```python
from build123d import *

# Parameters (mm, degrees)
SKETCH1_W           = 203.2
SKETCH1_H           = 101.6
BOSS_EXTRUDE2_DEPTH = 203.2
FILLET3_R           = 20
FILLET4_R           = 20
FILLET5_R           = 20
FILLET6_R           = 20
SKETCH2_W           = 152.4
SKETCH2_H           = 152.4
CUT_EXTRUDE1_DEPTH  = 88.9


with BuildPart() as part:
    # Sketch1 → Boss-Extrude2 (new body)
    with BuildSketch(Plane.XY):
        with Locations((101.6, 50.8)):
            Rectangle(SKETCH1_W, SKETCH1_H)
    extrude(amount=BOSS_EXTRUDE2_DEPTH)

    # Fillet3
    fillet3_edges = [part.edges().sort_by_distance(p)[0] for p in [
        (0, 50.8, 0),
    ]]
    fillet(fillet3_edges, radius=FILLET3_R)

    # Fillet4
    fillet4_edges = [part.edges().sort_by_distance(p)[0] for p in [
        (203.2, 50.8, 0),
    ]]
    fillet(fillet4_edges, radius=FILLET4_R)

    # Fillet5
    fillet5_edges = [part.edges().sort_by_distance(p)[0] for p in [
        (0, 50.8, 203.2),
    ]]
    fillet(fillet5_edges, radius=FILLET5_R)

    # Fillet6
    fillet6_edges = [part.edges().sort_by_distance(p)[0] for p in [
        (203.2, 50.8, 203.2),
    ]]
    fillet(fillet6_edges, radius=FILLET6_R)

    # Sketch2 → Cut-Extrude1 (cut)
    with BuildSketch(Plane.XZ):
        with Locations((100, 100)):
            Rectangle(SKETCH2_W, SKETCH2_H)
    extrude(amount=-CUT_EXTRUDE1_DEPTH, mode=Mode.SUBTRACT)


solid = part.part
```
Can you work these out from the model? Positions are in its coordinate system, mm. A direction names the side the tool comes from. Round coordinates to 2 decimals unless told otherwise and drop trailing zeros. Order: outer loops, then holes, each group sorted by start corner. A loop starts at its lowest first (then second) coordinate and runs counter-clockwise, first axis right, second up.
(1) If we section it at A-A (z = 52.5): Please give me the cut outline in (x, y), plus the area to 3 significant figures.
Results are:
outline: (0, 0) - (23.8, 0) - (23.8, 88.9) - (176.2, 88.9) - (176.2, 0) - (203.2, 0) - (203.2, 101.6) - (0, 101.6) - close
area: 7,100 mm2
(2) We'd pull the mould along Z, two halves only. Please class faces 1 (the face through (99, 44, 176.2)), 2 (the face through (5.703, 51.511, 6.014)), 3 (the face through (197.186, 51.511, 197.497)): +Z half, -Z half, draft (parallel to the pull), parting line (faces both ways), or undercut.
Results are:
face 1: undercut
face 2: -Z half
face 3: +Z half
(3) If we section it at C-C (y = 53): Please give me the cut outline in (x, z).
Results are:
outline: (0, 20) arc R20 ccw to (20, 0) - (183.2, 0) arc R20 ccw to (203.2, 20) - (203.2, 183.2) arc R20 ccw to (183.2, 203.2) - (20, 203.2) arc R20 ccw to (0, 183.2) - close; hole (23.8, 23.8) - (176.2, 23.8) - (176.2, 176.2) - (23.8, 176.2) - close
(4) If I drill on L1, parallel to X at y = 35, z = 30; L2, parallel to Y at x = 143.5, z = 30, over which ranges is the centre line in solid material (lowest first)?
Results are:
L1: x = 0 to 23.8, 176.2 to 203.2
L2: y = 88.9 to 101.6
(5) On a 3-axis mill with a long thin cutter (end or side, diameter ignored), from which of +Z, -Z, +X, -X, +Y, -Y can I reach the whole of each face in a straight line? I mean faces 4 (the face through (203.2, 50, 100)), 5 (the face through (99, 44, 23.8)). Say none if no direction works.
Results are:
face 4: +Z, -Z, +X, +Y, -Y
face 5: -Y
(6) If we section it at B-B (x = 61): Please give me the cut outline in (y, z), plus the area to 3 significant figures.
Results are:
outline: (0, 0) - (101.6, 0) - (101.6, 203.2) - (0, 203.2) - (0, 176.2) - (88.9, 176.2) - (88.9, 23.8) - (0, 23.8) - close
area: 7,100 mm2
